Source: CAD feature listing. Evaluate the final solid. Frame: model axes, mm. A direction names the side the tool comes from. Coordinates: 2 decimals unless noted, no trailing zeros. Write each loop counter-clockwise with the first axis right and the second up, starting at its lowest first coordinate (ties: lowest second). Pieces come first, ordered by that corner, then holes. Notation, with made-up numbers: (-6, 11) - (21, 11) arc R10 ccw to (21, 22) - close; hole circle Ø4 at (48.25, -2.5). An arc over 180 degrees is marked (long way). One line per item, written item: value.
from build123d import *

# Parameters (mm, degrees)
EXTRUDE2_DEPTH = 4.7
EXTRUDE3_DEPTH = 2.8


with BuildPart() as part:
    # Sketch1 → Extrude2 (new body)
    with BuildSketch(Plane(origin=(0, 0, 0), x_dir=(1, 0, 0), z_dir=(0, 1, 0))):
        with BuildLine():
            Line((0, 0), (30, 0))
            Line((30, 0), (30, 3))
            Line((30, 3), (27.428441876, 6.776441992))
            ThreePointArc((27.428441876, 6.776441992), (26.604060948, 8.988997747), (24.850416315, 10.570053529))
            ThreePointArc((24.850416315, 10.570053529), (24.500644991, 12.5), (24.850416315, 14.429946471))
            ThreePointArc((24.850416315, 14.429946471), (26.604060948, 16.011002253), (27.428441876, 18.223558008))
            Line((27.428441876, 18.223558008), (30, 22))
            Line((30, 22), (30, 25))
            Line((30, 25), (0, 25))
            Line((0, 25), (0, 22))
            Line((0, 22), (2.571558124, 18.223558008))
            ThreePointArc((2.571558124, 18.223558008), (3.395939052, 16.011002253), (5.149583685, 14.429946471))
            ThreePointArc((5.149583685, 14.429946471), (5.499355009, 12.5), (5.149583685, 10.570053529))
            ThreePointArc((5.149583685, 10.570053529), (3.395939052, 8.988997747), (2.571558124, 6.776441992))
            Line((2.571558124, 6.776441992), (0, 3))
            Line((0, 3), (0, 0))
        make_face()
    extrude(amount=EXTRUDE2_DEPTH)

    # Sketch3 → Extrude3 (add)
    with BuildSketch(Plane(origin=(0, 4.7, 0), x_dir=(1, 0, 0), z_dir=(0, 1, 0))):
        with BuildLine():
            Line((2.54, 6.2), (2.54, 0))
            Line((2.54, 0), (12.46, 0))
            Line((12.46, 0), (12.46, 6.2))
            ThreePointArc((12.46, 6.2), (7.5, 11.16), (2.54, 6.2))
        make_face()
        Polygon((7.5, 10.03), (4.183122704, 8.115), (4.183122704, 4.285), (7.5, 2.37), (10.816877296, 4.285), (10.816877296, 8.115), align=None, mode=Mode.SUBTRACT)
        with BuildLine():
            Line((2.54, 18.8), (2.54, 25))
            Line((2.54, 25), (12.46, 25))
            Line((12.46, 25), (12.46, 18.8))
            ThreePointArc((12.46, 18.8), (7.5, 13.84), (2.54, 18.8))
        make_face()
        Polygon((7.5, 22.63), (4.183122704, 20.715), (4.183122704, 16.885), (7.5, 14.97), (10.816877296, 16.885), (10.816877296, 20.715), align=None, mode=Mode.SUBTRACT)
        with BuildLine():
            Line((27.46, 0), (17.54, 0))
            Line((17.54, 0), (17.54, 6.2))
            ThreePointArc((17.54, 6.2), (22.5, 11.16), (27.46, 6.2))
            Line((27.46, 6.2), (27.46, 0))
        make_face()
        Polygon((19.183122704, 4.285), (19.183122704, 8.115), (22.5, 10.03), (25.816877296, 8.115), (25.816877296, 4.285), (22.5, 2.37), align=None, mode=Mode.SUBTRACT)
        with BuildLine():
            Line((17.54, 18.8), (17.54, 25))
            Line((17.54, 25), (27.46, 25))
            Line((27.46, 25), (27.46, 18.8))
            ThreePointArc((27.46, 18.8), (22.5, 13.84), (17.54, 18.8))
        make_face()
        Polygon((25.816877296, 16.885), (22.5, 14.97), (19.183122704, 16.885), (19.183122704, 20.715), (22.5, 22.63), (25.816877296, 20.715), align=None, mode=Mode.SUBTRACT)
    extrude(amount=EXTRUDE3_DEPTH)


solid = part.part
1) Reachability of faces 1 (the flat face through (5.865, 6.08, -21.686)), 2 (the flat face through (12.46, 6, -3)), 3 (the cylindrical face through (3.415, 2.317, -9.017)) from +Z, -Z, +X, -X, +Y, -Y: full face, straight path, thin tool, end or side. Return the list, or none.
Values found:
face 1: +Y
face 2: +Z, -Z, +Y
face 3: -X, +Y, -Y
2) Material intervals for line 1 (X direction, y = 5.5, z = -8.75); line 2 (Z direction, x = 21, y = 6.75); line 3 (Z direction, x = 4.75, y = 6.5), sorted ascending.
Values found:
line 1: 3.25 to 5.28, 9.72 to 11.75, 18.25 to 20.28, 24.72 to 26.75
line 2: -25 to -21.76, -15.84 to -14.07, -10.93 to -9.16, -3.24 to 0
line 3: -25 to -21.04, -16.56 to -14.67, -10.33 to -8.44, -3.96 to 0
3) Draft query along X for faces 4 (the cylindrical face through (22.39, 6.08, -11.16)), 5 (the flat face through (28.7, 2.32, -20.09)), 6 (the flat face through (15, 4, -25)). Return one class per face: released by +X, released by -X, zero draft, split by the parting line, or undercut.
Values found:
face 4: undercut
face 5: released by +X
face 6: zero draft
4) Section query C-C on y = 6.25. State how many separate pieces and enclosed holes the cut face has, then the cut area to 3 significant figures.
Values found:
separate pieces: 4
enclosed holes: 4
area: 248 mm2
5) Contact query for flat-ended pins moving along their axis: P1, Ø0.8, axis at y = 6, z = -2.5, coming from the -X side; P2, Ø2, axis at y = 6, z = -23, coming from the +X side; P3, Ø4, axis at y = 2.5, z = -7, coming from the +X side. Output: stop coordinate, or through.
Values found:
P1: x = 2.54
P2: x = 27.46
P3: x = 28.64
6) Section query A-A on y = 1. Output: boundary loops of the cut face in (x, z), then the cut area to 3 significant figures.
Values found:
outline: (0, -25) - (30, -25) - (30, -22) - (27.43, -18.22) arc R4.96 ccw to (24.85, -14.43) arc R5.5 cw to (24.85, -10.57) arc R4.96 ccw to (27.43, -6.78) - (30, -3) - (30, 0) - (0, 0) - (0, -3) - (2.57, -6.78) arc R4.96 ccw to (5.15, -10.57) arc R5.5 cw to (5.15, -14.43) arc R4.96 ccw to (2.57, -18.22) - (0, -22) - close
area: 637 mm2
